Autodesk Inventor part; units mm, degrees
ref_plane "YZ Plane" through (0, 0, 0) normal (1, 0, 0) x (0, 1, 0)
ref_plane "XZ Plane" through (0, 0, 0) normal (0, 1, 0) x (-1, 0, 0)
ref_plane "XY Plane" through (0, 0, 0) normal (0, 0, 1) x (1, 0, 0)
sketch "Skizze1" plane through (0, 0, 0) normal (0, 0, 1) x (1, 0, 0)
  line L0 (-7, 9.15) -> (7, 9.15)
  line L1 (7, 9.15) -> (7, -9.15)
  line L2 (7, -9.15) -> (-7, -9.15)
  line L3 (-7, -9.15) -> (-7, 9.15)
  line L4 (-7, 9.15) -> (7, -9.15) construction
  line L5 (7, 9.15) -> (-7, -9.15) construction
  point P0 (0, 0)
  dimension "d0" = 14
  dimension "d1" = 18.3
extrude "Extrusion1" add sketch "Skizze1" along normal blind 1.9
chamfer "Fasen1" distance 1.5 angle 45 4 edges at (-7, -9.15, 0.95) (7, -9.15, 0.95) (7, 9.15, 0.95) (-7, 9.15, 0.95)
sketch "Skizze2" plane through (0, 0, 1.9) normal (0, 0, 1) x (1, 0, 0)
  line L0 (7, -6) -> (-3, -6)
  line L1 (-3, -6) -> (-3, 6)
  line L2 (-3, 6) -> (7, 6)
  line L3 (7, 6) -> (7, -6)
  point P0 (0, 0)
  point P1 (7, 7.65)
  point P2 (-3, 0)
  dimension "d7" = 10
  dimension "d8" = 12
extrude "Extrusion2" add sketch "Skizze2" along normal blind 10
sketch "Skizze3" plane through (0, 0, 11.9) normal (0, 0, 1) x (1, 0, 0)
  line L0 (-17.5, 15) -> (17.5, 15)
  line L1 (17.5, 15) -> (17.5, -15)
  line L2 (17.5, -15) -> (-17.5, -15)
  line L3 (-17.5, -15) -> (-17.5, 15)
  line L4 (-17.5, 15) -> (17.5, -15) construction
  line L5 (17.5, 15) -> (-17.5, -15) construction
  point P0 (0, 0)
  dimension "d11" = 35
  dimension "d12" = 30
extrude "Extrusion3" add sketch "Skizze3" along normal blind 3
sketch "Skizze4" plane through (0, 0, 11.9) normal (0, 0, -1) x (-1, 0, 0)
  line L0 (12.5, -10) -> (-12.5, -10)
  line L1 (-12.5, -10) -> (-12.5, 10)
  line L2 (-12.5, 10) -> (12.5, 10)
  line L3 (12.5, 10) -> (12.5, -10)
  line L4 (12.5, -10) -> (-12.5, 10) construction
  line L5 (-12.5, -10) -> (12.5, 10) construction
  point P0 (0, 0)
  dimension "d15" = 25
  dimension "d16" = 20
hole "Bohrung1" at (-12.5, -10, 11.9) at (12.5, 10, 11.9) direction (0, 0, 1) diameter 4.2 end through all
fillet "Rundung1" radius 5 1 edges at (-3, 0, 11.9)
fillet "Rundung2" radius 3 3 edges at (2, -6, 11.9) (2, 6, 11.9) (7, 0, 11.9)
fillet "Rundung3" radius 3 4 edges at (-17.5, -15, 13.4) (-17.5, 15, 13.4) (17.5, 15, 13.4) (17.5, -15, 13.4)
properties part number "hotshouh mount"
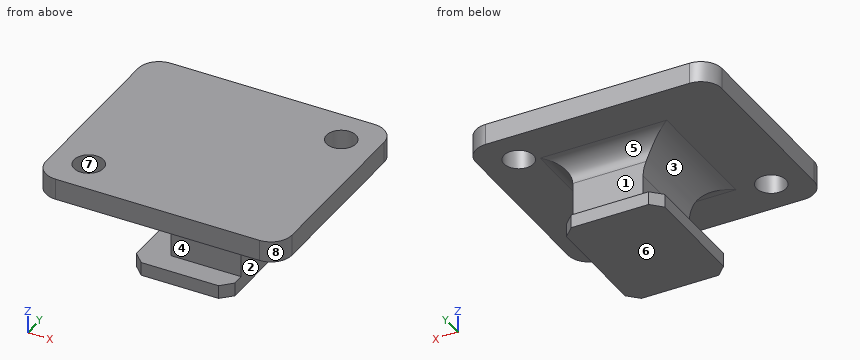
Here's how the part is built. I have some questions about the finished solid (model axes, mm). Face numbers are marked on the shaded views. A direction names the side the tool comes from. Round coordinates to 2 decimals unless told otherwise and drop trailing zeros. Write each loop counter-clockwise with the first axis right and the second up, starting at its lowest first coordinate (ties: lowest second). Pieces come first, ordered by that corner, then holes.
Q1. If we mould it in two halves opening along Y, with no side actions, what happens to the marked faces 5, 6, 7 and 8? For each: +Y half, -Y half, draft (parallel to the pull), parting line (faces both ways), or undercut.
Q2. If we section it at C-C on z = 14: Write out the boundary of the cut face in (x, y), plus the area to 3 significant figures.
Q3. Will these pins go through, and if not, where does the flat tip stop? P1, Ø4, axis at y = -3, z = 4.5, coming from the -X side; P2, Ø5, axis at x = 12.5, y = 10, coming from the -Z side; P3, Ø3, axis at x = 0.5, y = 0.5, coming from the -Z side; P4, Ø3.5, axis at x = 0.5, z = 6.5, coming from the -Y side.
Q4. If we section it at D-D on y = 3.25: Write out the boundary of the cut face in (x, z), plus the area to 3 significant figures.
Q5. Please list where these lines run through material, in increasing order: probe 1 along Y at (x, z) = (-12.5, 13.9); probe 2 along Y at (x, z) = (12.5, 13.8); probe 3 along X at (y, z) = (-10, 14.35).
Q6. If we section it at B-B on y = -10: Write out the boundary of the cut face in (x, z), plus the area to 3 significant figures.
Q7. Which directions (+Z, -Z, +X, -X, +Y, -Y) give clear straight access to the entire face, cutting with the end or side of a thin tool? Please do the marked faces 1, 2, 3 and 4.
Q8. If we section it at A-A on x = -12.5: Write out the boundary of the cut face in (y, z), plus the area to 3 significant figures.
Answer below:
1. face 5: +Y half
1. face 6: draft
1. face 7: undercut
1. face 8: -Y half
2. outline: (-17.5, -12) arc R3 ccw to (-14.5, -15) - (14.5, -15) arc R3 ccw to (17.5, -12) - (17.5, 12) arc R3 ccw to (14.5, 15) - (-14.5, 15) arc R3 ccw to (-17.5, 12) - close; hole circle Ø4.2 at (-12.5, -10); hole circle Ø4.2 at (12.5, 10)
2. area: 1,010 mm2
3. P1: stops at x = -3
3. P2: stops at z = 11.9
3. P3: stops at z = 0
3. P4: stops at y = -6
4. outline: (-17.5, 11.9) - (-8, 11.9) arc R5 cw to (-3, 6.9) - (-3, 1.9) - (-7, 1.9) - (-7, 0) - (7, 0) - (7, 8.9) arc R3 cw to (10, 11.9) - (17.5, 11.9) - (17.5, 14.9) - (-17.5, 14.9) - close
4. area: 239 mm2
5. probe 1: y = -15 to -12.1, -7.9 to 15
5. probe 2: y = -15 to 7.9, 12.1 to 15
5. probe 3: x = -17.5 to -14.6, -10.4 to 17.5
6. outline: (-17.5, 11.9) - (-14.6, 11.9) - (-14.6, 14.9) - (-17.5, 14.9) - close; (-10.4, 11.9) - (17.5, 11.9) - (17.5, 14.9) - (-10.4, 14.9) - close
6. area: 92.4 mm2
7. face 1: +X, -X, +Y
7. face 2: -Z, +X, +Y, -Y
7. face 3: -X, +Y, -Y
7. face 4: +X, -X, -Y
8. outline: (-15, 11.9) - (-12.1, 11.9) - (-12.1, 14.9) - (-15, 14.9) - close; (-7.9, 11.9) - (15, 11.9) - (15, 14.9) - (-7.9, 14.9) - close
8. area: 77.4 mm2
